The model under review builds one solid part; all positions refer to its coordinate system, in mm. A direction names the side the tool comes from. Coordinates: 2 decimals unless noted, no trailing zeros. Loops run counter-clockwise (first coordinate to the right, second up) from the corner with the lowest first, then second, coordinate; pieces in that order, holes last. Notation, with made-up numbers: (-28, 62.25) - (-23, 62.25) arc R25 cw to (-23, 81.25) - close; hole circle Ø6 at (58.25, 61). An arc over 180 degrees is marked (long way). Answer in a Markdown table with one row per item. Add a question column.
(1) We need section C-C on y = 3.25. Write out the cut boundary in (x, z).
(2) For line 1 along Z through (x, y) = (7.5, 12.75); line 2 along X through (y, z) = (-1, -7.5); line 3 along Y through (x, z) = (52, -18.8), list the stretches that pass through material, from the lowest coordinate up.
(3) Machinability: for faces 4 (the flat face through (-1, 8, 18.2)), 5 (the flat face through (0, -1, 4.5)), 6 (the flat face through (-35, 0, 19)), 7 (the flat face through (43, 1.758, 19)), which of the approach directions +Z, -Z, +X, -X, +Y, -Y give a long, thin tool a straight path to every point of the face, cutting with its end or side? Answer none if there is none.
(4) Mouldability with a two-part tool opening along X and no side actions: class faces 1 (the cylindrical face through (-0.542, 10.817, -19.186)), 2 (the flat face through (56, -1, 0)), 3 (the flat face through (1, 0, 0)) as +X half, -X half, draft (parallel to the pull), parting line (faces both ways), or undercut.
(5) We need section D-D on z = -1.5. Write out the cut boundary in (x, y).
(6) We need section B-B on x = 10.5. Write out the cut boundary in (y, z).
(7) For P1, Ø1, axis at x = 43, y = -1.5, coming from the -Z side; P2, Ø1, axis at x = 44, z = -19, coming from the -Y side; P3, Ø1.5, axis at x = -52, y = 5.76, coming from the -Z side; P4, Ø2, axis at x = 9, y = -1, coming from the +Z side, all flat-tipped, find the tip position at first contact; note any pin that passes through.
(8) We need section A-A on x = -38. Write out the cut boundary in (y, z), plus the area to 3 significant figures.
from build123d import *

# Parameters (mm, degrees)
BRIDA_BASE1_DEPTH               = 2
PLIEGUE_START                   = -56
PLIEGUE_CROQUIZADO2_DEPTH       = 112
PLIEGUE_CROQUIZADO2_2_OUTLINE_W = 19
PLIEGUE_CROQUIZADO2_2_OUTLINE_H = 2
PLIEGUE_CROQUIZADO2_2_DEPTH     = 112
PLIEGUE_START_2                 = -35
PLIEGUE_CROQUIZADO2_3_DEPTH     = 70
CROQUIS10_R                     = 1.25
CROQUIS10_R_2                   = 2.5
CORTAR_EXTRUIR2_DEPTH           = 73.104459651
CROQUIS11_R                     = 1.25
CORTAR_EXTRUIR3_DEPTH           = 10
REDONDEO1_R                     = 10


# Read off the part's stored shape, not the designer's step: Pliegue croquizado2
# Sheet-metal steps are written as plain solids
with BuildPart() as part:
    # Croquis base → Brida base1 (new body)
    with BuildSketch(Plane(origin=(0, 0, 0), x_dir=(1, 0, 0), z_dir=(0, 1, 0))):
        Polygon((56, 17.9), (56, -17.9), (35, -17.9), (35, -21.4), (56, -21.4), (56, -40.4), (-56, -40.4), (-56, -21.4), (-35, -21.4), (-35, -17.9), (-56, -17.9), (-56, 17.9), (-35, 17.9), (-35, 21.4), (-56, 21.4), (-56, 40.4), (56, 40.4), (56, 21.4), (35, 21.4), (35, 17.9), align=None)
    extrude(amount=-BRIDA_BASE1_DEPTH)

    # Pliegue croquizado2 outline → Pliegue croquizado2 (cut)
    with BuildSketch(Plane.YZ.offset(PLIEGUE_START)):
        with BuildLine():
            ThreePointArc((0, -20.18035085), (-1.429161647, -19.416575089), (-2, -17.9))
            Line((-2, -17.9), (-2, -40.4))
            Line((-2, -40.4), (0, -40.4))
            Line((0, -40.4), (0, -20.18035085))
        make_face()
        with BuildLine():
            ThreePointArc((-2, 17.9), (-1.429161647, 19.416575089), (0, 20.18035085))
            Line((0, 20.18035085), (0, 40.4))
            Line((0, 40.4), (-2, 40.4))
            Line((-2, 40.4), (-2, 17.9))
        make_face()
    extrude(amount=PLIEGUE_CROQUIZADO2_DEPTH, mode=Mode.SUBTRACT)



with BuildPart() as body_2:
    # Pliegue croquizado2 2 outline → Pliegue croquizado2 2 (new body)
    with BuildSketch(Plane.YZ.offset(PLIEGUE_START)):
        with Locations((11.257964775, -19.2)):
            Rectangle(PLIEGUE_CROQUIZADO2_2_OUTLINE_W, PLIEGUE_CROQUIZADO2_2_OUTLINE_H)
        with Locations((11.257964775, 19.2)):
            Rectangle(PLIEGUE_CROQUIZADO2_2_OUTLINE_W, PLIEGUE_CROQUIZADO2_2_OUTLINE_H)
    extrude(amount=PLIEGUE_CROQUIZADO2_2_DEPTH)


with BuildPart() as part_1:
    add(part.part)

    add(body_2.part)  # Pliegue croquizado2 3 merges body 2
    # Pliegue croquizado2 3 outline → Pliegue croquizado2 3 (add)
    with BuildSketch(Plane.YZ.offset(PLIEGUE_START_2)):
        with BuildLine():
            Line((0, -17.9), (0, -20.18035085))
            ThreePointArc((0, -20.18035085), (0.149678603, -20.195082456), (0.3, -20.2))
            Line((0.3, -20.2), (1.757964775, -20.2))
            Line((1.757964775, -20.2), (1.757964775, -18.2))
            Line((1.757964775, -18.2), (0.3, -18.2))
            ThreePointArc((0.3, -18.2), (0.087867966, -18.112132034), (0, -17.9))
        make_face()
        with BuildLine():
            ThreePointArc((0.3, 20.2), (0.149678603, 20.195082456), (0, 20.18035085))
            Line((0, 20.18035085), (0, 17.9))
            ThreePointArc((0, 17.9), (0.087867966, 18.112132034), (0.3, 18.2))
            Line((0.3, 18.2), (1.757964775, 18.2))
            Line((1.757964775, 18.2), (1.757964775, 20.2))
            Line((1.757964775, 20.2), (0.3, 20.2))
        make_face()
    extrude(amount=PLIEGUE_CROQUIZADO2_3_DEPTH)

    # Croquis10 → Cortar-Extruir2 (cut, through all)
    with BuildSketch(Plane.XY.offset(20.2)):
        with BuildLine():
            ThreePointArc((-56, 5.757964775), (-54.828427125, 8.5863919), (-52, 9.757964775))
            Line((-52, 9.757964775), (-25, 9.757964775))
            Line((-25, 9.757964775), (-3.19965236, 20.041195921))
            ThreePointArc((-3.19965236, 20.041195921), (-1.639476503, 20.576579179), (0, 20.757964775))
            Line((0, 20.757964775), (-56, 20.757964775))
            Line((-56, 20.757964775), (-56, 5.757964775))
        make_face()
        with BuildLine():
            ThreePointArc((-52, 1.757964775), (-54.828427125, 2.92953765), (-56, 5.757964775))
            Line((-56, 5.757964775), (-56, 1.757964775))
            Line((-56, 1.757964775), (-52, 1.757964775))
        make_face()
        with BuildLine():
            Line((56, 20.757964775), (0, 20.757964775))
            ThreePointArc((0, 20.757964775), (1.639476503, 20.576579179), (3.19965236, 20.041195921))
            Line((3.19965236, 20.041195921), (25, 9.757964775))
            Line((25, 9.757964775), (52, 9.757964775))
            ThreePointArc((52, 9.757964775), (54.828427125, 8.5863919), (56, 5.757964775))
            Line((56, 5.757964775), (56, 20.757964775))
        make_face()
        with BuildLine():
            Line((56, 1.757964775), (56, 5.757964775))
            ThreePointArc((56, 5.757964775), (54.828427125, 2.92953765), (52, 1.757964775))
            Line((52, 1.757964775), (56, 1.757964775))
        make_face()
        with Locations((52, 5.757964775)):
            Circle(CROQUIS10_R)
        with Locations((10.5, 9.357964775)):
            Circle(CROQUIS10_R)
        with Locations((-10.5, 9.357964775)):
            Circle(CROQUIS10_R)
        with Locations((0, 13.257964775)):
            Circle(CROQUIS10_R_2)
        with Locations((-52, 5.757964775)):
            Circle(CROQUIS10_R)
    extrude(amount=-CORTAR_EXTRUIR2_DEPTH, mode=Mode.SUBTRACT)

    # Croquis11 → Cortar-Extruir3 (cut)
    with BuildSketch(Plane(origin=(0, 0, 0), x_dir=(1, 0, 0), z_dir=(0, 1, 0))):
        with Locations(Location((-50, 7.5, 0), (0, 0, 270))):
            Circle(CROQUIS11_R)
        with Locations(Location((50, 7.5, 0), (0, 0, 270))):
            Circle(CROQUIS11_R)
        with Locations(Location((50, -7.5, 0), (0, 0, 90))):
            Circle(CROQUIS11_R)
        with Locations(Location((-50, -7.5, 0), (0, 0, 90))):
            Circle(CROQUIS11_R)
        with BuildLine():
            Line((-22.5, 10.5), (22.5, 10.5))
            ThreePointArc((22.5, 10.5), (25.5, 7.5), (22.5, 4.5))
            Line((22.5, 4.5), (-22.5, 4.5))
            ThreePointArc((-22.5, 4.5), (-25.5, 7.5), (-22.5, 10.5))
        make_face()
        with BuildLine():
            Line((-22.5, -10.5), (22.5, -10.5))
            ThreePointArc((22.5, -10.5), (25.5, -7.5), (22.5, -4.5))
            Line((22.5, -4.5), (-22.5, -4.5))
            ThreePointArc((-22.5, -4.5), (-25.5, -7.5), (-22.5, -10.5))
        make_face()
    extrude(amount=-CORTAR_EXTRUIR3_DEPTH, mode=Mode.SUBTRACT)

    # Redondeo1
    redondeo1_edges = [part_1.edges().sort_by_distance(p)[0] for p in [
        (-56, -1, 17.9),
        (-56, -1, -17.9),
        (56, -1, -17.9),
        (56, -1, 17.9),
    ]]
    fillet(redondeo1_edges, radius=REDONDEO1_R)


solid = part_1.part
Outcome:
| question | item | result |
|---|---|---|
| 1 | outline | (-55.12, -20.2) - (55.12, -20.2) - (55.12, -18.2) - (-55.12, -18.2) - close; (-55.12, 18.2) - (55.12, 18.2) - (55.12, 20.2) - (-55.12, 20.2) - close |
| 2 | line 1 | -20.2 to -18.2, 18.2 to 20.2 |
| 2 | line 2 | -56 to -51.25, -48.75 to -25.5, 25.5 to 48.75, 51.25 to 56 |
| 2 | line 3 | 1.76 to 4.51, 7.01 to 9.76 |
| 3 | face 4 | +X, -X, +Y |
| 3 | face 5 | +Y, -Y |
| 3 | face 6 | +Z, -X, -Y |
| 3 | face 7 | +Z, -Z, +X, -Y |
| 4 | face 1 | undercut |
| 4 | face 2 | +X half |
| 4 | face 3 | draft |
| 5 | outline | (-56, -2) - (56, -2) - (56, 0) - (-56, 0) - close |
| 6 | outline | (-2, -17.9) arc R2.3 ccw to (0.3, -20.2) - (8.11, -20.2) - (8.11, -18.2) - (0.3, -18.2) arc R0.3 cw to (0, -17.9) - (0, -10.5) - (-2, -10.5) - close; (-2, -4.5) - (0, -4.5) - (0, 4.5) - (-2, 4.5) - close; (-2, 10.5) - (0, 10.5) - (0, 17.9) arc R0.3 cw to (0.3, 18.2) - (8.11, 18.2) - (8.11, 20.2) - (0.3, 20.2) arc R2.3 ccw to (-2, 17.9) - close; (10.61, -20.2) - (16.6, -20.2) - (16.6, -18.2) - (10.61, -18.2) - close; (10.61, 18.2) - (16.6, 18.2) - (16.6, 20.2) - (10.61, 20.2) - close |
| 7 | P1 | z = -17.9 |
| 7 | P2 | y = 1.76 |
| 7 | P3 | through |
| 7 | P4 | z = 20.18 |
| 8 | outline | (-2, -17.9) - (0, -17.9) - (0, 17.9) - (-2, 17.9) - close; (1.76, -20.2) - (9.76, -20.2) - (9.76, -18.2) - (1.76, -18.2) - close; (1.76, 18.2) - (9.76, 18.2) - (9.76, 20.2) - (1.76, 20.2) - close |
| 8 | area | 104 mm² |
